Check sheet for the modelled part. Datum: model origin and axes. Units: mm. Face numbers are marked on the shaded views. Give positions to 0.01 mm unless a question says otherwise; leave off trailing zeros. Write each loop counter-clockwise with the first axis right and the second up, starting at its lowest first coordinate (ties: lowest second). Pieces come first, ordered by that corner, then holes. Notation, with made-up numbers: M 30.5,-37 L 57.5,-37 A10 cw 57.5,-18 Z; hole C 70,64.5 d9. An arc over 180 degrees is marked long. Write item = value, one per line. Start each with the question number.
1) Mould release check, pull along Z, two halves, no side actions. Record for the marked faces 1, 2, 3 and 4: released by +Z, released by -Z, zero draft, split by the parting line, or undercut.
2) Scan lines: line 1 along Z through (x, y) = (0, 0.45); line 2 along X through (y, z) = (0.55, 0.45). Record each from-to range of solid material in increasing order. Write a range as [from, to].
3) Cross-section at D-D, the plane x = -1.2. Record the cut outline in (y, z).
4) Cross-section at C-C, the plane y = 1.75. Record the cut outline in (x, z), plus the area to 3 significant figures.
5) Go/stop test with flat-tipped pins: pin 1 (1.5 mm diameter, centred on y = 0.5, z = -1, fed in from +X); pin 2 (1 mm diameter, centred on y = 1, z = 1, fed in from -X). Record where each tip stops, or that it passes through.
6) Cross-section at A-A, the plane x = 0. Record the cut outline in (y, z), plus the area to 3 significant figures.
7) Cross-section at B-B, the plane z = -0.7. Record the cut outline in (x, y), plus the area to 3 significant figures.
Autodesk Inventor part; units mm, degrees
ref_plane "YZ Plane" through (0, 0, 0) normal (1, 0, 0) x (0, 1, 0)
ref_plane "XZ Plane" through (0, 0, 0) normal (0, 1, 0) x (-1, 0, 0)
ref_plane "XY Plane" through (0, 0, 0) normal (0, 0, 1) x (1, 0, 0)
sketch "Sketch1" plane through (0, 0, 0) normal (0, 1, 0) x (-1, 0, 0)
  circle A0 centre (0, 0) radius 2.25
  circle A1 centre (0, 0) radius 1.9
  dimension "d0" = 4.5
  dimension "d1" = 3.8
extrude "Extrusion1" add sketch "Sketch1" along normal blind 0.96
sketch "Sketch2" plane through (0, 0, 0) normal (1, 0, 0) x (0, 1, 0)
  arc A0 (0.96, -3) -> (0.96, 3) centre (-0.29, 0) ccw
  line L0 (0.96, -2.25) -> (0.96, 2.25)
  line L1 (0.96, 3) -> (0.96, 2.25)
  line L2 (0.96, -3) -> (0.96, -2.25)
  line L3 (2.96, 0) -> (0.96, 0)
  point P0 (0, 0)
  dimension "d4" = 2
  dimension "d5" = 3
revolve "Revolution1" add sketch "Sketch2" angle 360 about axis through (0, 2.96, 0) along (0, -1, 0) contours L3 L0 L1 A0
sketch "Sketch3" plane through (0, 0.96, 0) normal (0, -1, 0) x (1, 0, 0)
  line L0 (-2.25, 1) -> (2.25, 1)
  line L1 (2.25, 1) -> (2.25, -1)
  line L2 (2.25, -1) -> (-2.25, -1)
  line L3 (-2.25, -1) -> (-2.25, 1)
  line L4 (-2.25, 1) -> (2.25, -1) construction
  line L5 (2.25, 1) -> (-2.25, -1) construction
  circle A0 centre (0, 0) radius 2.25
  circle A1 centre (0, 0) radius 1.9
  point P0 (1.6155, 1)
  point P1 (-1.6155, 1)
  point P2 (-1.6155, -1)
  point P3 (1.6155, -1)
  dimension "d7" = 2
extrude "Extrusion2" cut sketch "Sketch3" against normal blind 0.16 contours L0 A1 L2
properties part number "Hephaestus38v2 Case Feet" material "Thermoplastic Resin"
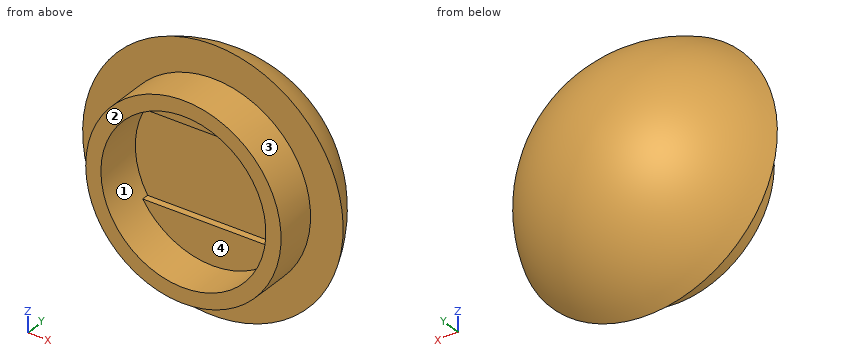
Reply:
q1.face_1 = undercut
q1.face_2 = zero draft
q1.face_3 = split by the parting line
q1.face_4 = undercut
q2.line_1 = [-2.25, -1.9], [1.9, 2.25]
q2.line_2 = [-2.2, -1.85], [1.85, 2.2]
q3.outline = M 0,-1.9 L 0.96,-1.9 L 0.96,-2.75 A3.02 ccw 0.96,2.75 L 0.96,1.9 L 0,1.9 L 0,1.47 L 0.96,1.47 L 0.96,1 L 1.12,1 L 1.12,-1 L 0.96,-1 L 0.96,-1.47 L 0,-1.47 Z
q4.outline = C 0,0 d5.06
q4.area = 20.1 mm2
q5.pin_1 = 2.97
q5.pin_2 = -2.96
q6.outline = M 0,-2.25 L 0.96,-2.25 L 0.96,-3 A3.25 ccw 0.96,3 L 0.96,2.25 L 0,2.25 L 0,1.9 L 0.96,1.9 L 0.96,1 L 1.12,1 L 1.12,-1 L 0.96,-1 L 0.96,-1.9 L 0,-1.9 Z
q6.area = 9.02 mm2
q7.outline = M -2.92,0.96 L -2.14,0.96 L -2.14,0 L -1.77,0 L -1.77,1.12 L 1.77,1.12 L 1.77,0 L 2.14,0 L 2.14,0.96 L 2.92,0.96 A3.17 ccw Z
q7.area = 8.25 mm2
